Design review of the part built by this model. Coordinates are the model's own, in mm. Face numbers are marked on the shaded views. A direction names the side the tool comes from. Give positions to 0.01 mm unless a question says otherwise; leave off trailing zeros. Write each loop counter-clockwise with the first axis right and the second up, starting at its lowest first coordinate (ties: lowest second). Pieces come first, ordered by that corner, then holes. Notation, with made-up numbers: M 85,-40 L 96,-40 A22 cw 96,-15 Z; hole C 75.5,76.25 d10. An arc over 180 degrees is marked long. Use one line per item in the form item = value. Start each with the question number.
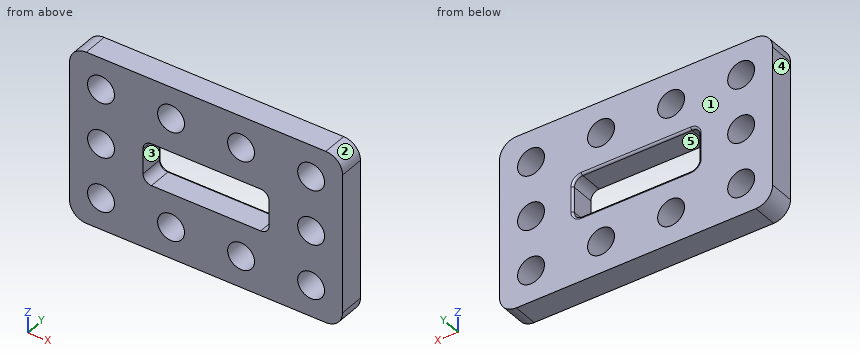
from build123d import *

# Parameters (mm, degrees)
F0_W     = 32.5
F0_H     = 20.5
F0_W_2   = 15
F0_H_2   = 5
F1_DEPTH = 3
F2_R     = 1.6
F3_DEPTH = 25
F4_R     = 1
F5_R     = 0.25
F6_R     = 2


with BuildPart() as f1:
    # F0 (on Front) → F1 (new body)
    with BuildSketch(Plane.XZ):
        with Locations((16.25, 10.25)):
            Rectangle(F0_W, F0_H)
        with Locations((16.25, 10.25)):
            Rectangle(F0_W_2, F0_H_2, mode=Mode.SUBTRACT)
    extrude(amount=F1_DEPTH)

    # F2 (on face) → F3 (cut)
    with BuildSketch(Plane.XZ.offset(3)):
        with Locations((3.75, 16.75)):
            Circle(F2_R)
        with Locations((3.75, 10.25)):
            Circle(F2_R)
        with Locations((3.75, 3.75)):
            Circle(F2_R)
        with Locations((12.0833333333, 16.75)):
            Circle(F2_R)
        with Locations((12.0833333333, 10.25)):
            Circle(F2_R)
        with Locations((12.0833333333, 3.75)):
            Circle(F2_R)
        with Locations((20.4166666667, 16.75)):
            Circle(F2_R)
        with Locations((20.4166666667, 10.25)):
            Circle(F2_R)
        with Locations((20.4166666667, 3.75)):
            Circle(F2_R)
        with Locations((28.75, 16.75)):
            Circle(F2_R)
        with Locations((28.75, 10.25)):
            Circle(F2_R)
        with Locations((28.75, 3.75)):
            Circle(F2_R)
    extrude(amount=-F3_DEPTH, mode=Mode.SUBTRACT)

    # F4
    f4_edges = [f1.edges().sort_by_distance(p)[0] for p in [
        (8.75, -1.5, 7.75),
        (8.75, -1.5, 12.75),
        (23.75, -1.5, 12.75),
        (23.75, -1.5, 7.75),
    ]]
    fillet(f4_edges, radius=F4_R)

    # F5
    f5_edges = [f1.edges().sort_by_distance(p)[0] for p in [
        (16.25, 0, 12.75),
        (9.042893, 0, 12.457107),
        (8.75, 0, 10.25),
        (9.042893, 0, 8.042893),
        (16.25, 0, 7.75),
        (23.457107, 0, 8.042893),
        (23.75, 0, 10.25),
        (23.457107, 0, 12.457107),
    ]]
    fillet(f5_edges, radius=F5_R)

    # F6
    f6_edges = [f1.edges().sort_by_distance(p)[0] for p in [
        (32.5, -1.5, 20.5),
        (32.5, -1.5, 0),
        (0, -1.5, 0),
        (0, -1.5, 20.5),
    ]]
    fillet(f6_edges, radius=F6_R)


solid = f1.part
1. Draft analysis for pull direction X (two halves, no side actions). For the marked faces 1, 2 and 3, state which applies: pulls with the +X half, pulls with the -X half, needs draft (parallel to the pull), parting line crosses it, or undercut.
2. We need section D-D (x = 28.75). State the section outline as (y, z) points, and give its area (3 significant figures).
3. Clearance check with flat-ended pins moving along their axes: pin 1 Ø3.5 at (x, z) = (28.75, 3.75) entering from -Y; pin 2 Ø3 at (x, z) = (12.08, 16.75) entering from +Y. State where each tip first meets the part, or that it passes through.
4. We need section C-C (z = 16.75). State the section outline as (x, y) points.
5. We need section A-A (z = 10.25). State the section outline as (x, y) points, and give its area (3 significant figures).
6. For the marked faces 4 and 5, list the 3-axis set-ups (+Z, -Z, +X, -X, +Y, -Y) from which the entire face can be reached by the end or side of a thin tool; tool diameter is ignored.
7. To check wall thickness, follow L1, parallel to Z at x = 20.5, y = -1.9; L2, parallel to Z at x = 28.75, y = -2.3; L3, parallel to Z at x = 18, y = -0.2. State the ranges of each line that lie inside material, in increasing order.
8. We need section B-B (x = 15.5). State the section outline as (y, z) points.
Answer block:
q1.face_1 = needs draft
q1.face_2 = pulls with the +X half
q1.face_3 = undercut
q2.outline = M -3,0 L 0,0 L 0,2.15 L -3,2.15 Z; M -3,5.35 L 0,5.35 L 0,8.65 L -3,8.65 Z; M -3,11.85 L 0,11.85 L 0,15.15 L -3,15.15 Z; M -3,18.35 L 0,18.35 L 0,20.5 L -3,20.5 Z
q2.area = 32.7 mm^2
q3.pin_1 = -3
q3.pin_2 = through
q4.outline = M 0,-3 L 2.15,-3 L 2.15,0 L 0,0 Z; M 5.35,-3 L 10.48,-3 L 10.48,0 L 5.35,0 Z; M 13.68,-3 L 18.82,-3 L 18.82,0 L 13.68,0 Z; M 22.02,-3 L 27.15,-3 L 27.15,0 L 22.02,0 Z; M 30.35,-3 L 32.5,-3 L 32.5,0 L 30.35,0 Z
q5.outline = M 0,-3 L 2.15,-3 L 2.15,0 L 0,0 Z; M 5.35,-3 L 8.75,-3 L 8.75,-0.25 A0.25 ccw 8.5,0 L 5.35,0 Z; M 23.75,-3 L 27.15,-3 L 27.15,0 L 24,0 A0.25 ccw 23.75,-0.25 Z; M 30.35,-3 L 32.5,-3 L 32.5,0 L 30.35,0 Z
q5.area = 33.3 mm^2
q6.face_4 = +Z, -Z, -X, +Y, -Y
q6.face_5 = +Y, -Y
q7.L1 = 0 to 2.15, 5.35 to 7.75, 12.75 to 15.15, 18.35 to 20.5
q7.L2 = 0 to 2.15, 5.35 to 8.65, 11.85 to 15.15, 18.35 to 20.5
q7.L3 = 0 to 7.74, 12.76 to 20.5
q8.outline = M -3,0 L 0,0 L 0,7.5 A0.25 ccw -0.25,7.75 L -3,7.75 Z; M -3,12.75 L -0.25,12.75 A0.25 ccw 0,13 L 0,20.5 L -3,20.5 Z
